```python
from build123d import *

# Parameters (mm, degrees)
SKETCH1_R                = 6
BOSS_EXTRUDE1_DEPTH      = 254
BOSS_EXTRUDE1_DEPTH_BACK = 36
CUT_EXTRUDE3_START       = -36
SKETCH2_W                = 4
SKETCH2_H                = 5
CUT_EXTRUDE3_DEPTH       = 20
CUT_EXTRUDE3_DEPTH_BACK  = 0.0001
CUT_EXTRUDE4_START       = 254
SKETCH2_2_W              = 4
SKETCH2_2_H              = 5
CUT_EXTRUDE4_DEPTH       = 50
CUT_EXTRUDE6_START       = -36
SKETCH3_W                = 4
SKETCH3_H                = 10
CUT_EXTRUDE6_DEPTH       = 6


with BuildPart() as part:
    # Sketch1 → Boss-Extrude1 (new body, two sides)
    with BuildSketch(Plane(origin=(0, 0, 0), x_dir=(1, 0, 0), z_dir=(0, 1, 0))) as boss_extrude1_sk:
        Circle(SKETCH1_R)
    extrude(amount=BOSS_EXTRUDE1_DEPTH)
    extrude(boss_extrude1_sk.sketch, amount=-BOSS_EXTRUDE1_DEPTH_BACK)

    # Sketch2 → Cut-Extrude3 (cut, two sides)
    with BuildSketch(Plane(origin=(0, 0, 0), x_dir=(1, 0, 0), z_dir=(0, 1, 0)).offset(CUT_EXTRUDE3_START)) as cut_extrude3_sk:
        with Locations((0, -6)):
            Rectangle(SKETCH2_W, SKETCH2_H)
    extrude(amount=CUT_EXTRUDE3_DEPTH, mode=Mode.SUBTRACT)
    extrude(cut_extrude3_sk.sketch, amount=-CUT_EXTRUDE3_DEPTH_BACK, mode=Mode.SUBTRACT)

    # Sketch2<2> → Cut-Extrude4 (cut)
    with BuildSketch(Plane(origin=(0, 0, 0), x_dir=(1, 0, 0), z_dir=(0, 1, 0)).offset(CUT_EXTRUDE4_START)):
        with Locations((0, -6)):
            Rectangle(SKETCH2_2_W, SKETCH2_2_H)
    extrude(amount=-CUT_EXTRUDE4_DEPTH, mode=Mode.SUBTRACT)

    # Sketch3 → Cut-Extrude6 (cut)
    with BuildSketch(Plane(origin=(0, 0, 0), x_dir=(1, 0, 0), z_dir=(0, 1, 0)).offset(CUT_EXTRUDE6_START)):
        with Locations((0, -6)):
            Rectangle(SKETCH3_W, SKETCH3_H)
    extrude(amount=CUT_EXTRUDE6_DEPTH, mode=Mode.SUBTRACT)


solid = part.part
```
Geometry check sheet. Reference: the model listing, model coordinates, mm. A direction names the side the tool comes from. Round coordinates to 2 decimals unless told otherwise and drop trailing zeros. Loops run counter-clockwise (first coordinate to the right, second up) from the corner with the lowest first, then second, coordinate; pieces in that order, holes last. Notation, with made-up numbers: (34, 73.5) - (80, 73.5) arc R19 ccw to (80, 96.5) - close; hole circle Ø11 at (37, 14). An arc over 180 degrees is marked (long way). Write each question's results on one line, items separated by ' | '. Start each with the question number.
Q1. Gauge pin test, flat ends, axial feed: P1, Ø1.1, axis at y = 224.5, z = 4, coming from the +X side; P2, Ø3, axis at x = 2.5, y = 34, coming from the -Z side; P3, Ø4.5, axis at x = 0, y = -25, coming from the +Z side. Record the tip position at first contact, or that the pin passes through.
Q2. Release check for a two-part mould opening along X. For faces 1 (the flat face through (2, -28, 4)), 2 (the flat face through (0, -36, 0)), 3 (the cylindrical face through (-0.78, 111.03, -5.95)) record: +X half, -X half, draft (parallel to the pull), parting line (faces both ways), or undercut.
Q3. Cross-section at C-C on y = 127. Enter the section's corners in (x, z), and give its area (3 significant figures).
Q4. Cross-section at A-A on x = 0. Enter the section's corners in (y, z), and give its area (3 significant figures).
Q5. Thickness scan on line 1 (Z direction, x = -0.25, y = 169.5); line 2 (Y direction, x = 0.5, z = 4.75); line 3 (X direction, y = 54.5, z = -0.75). Record the ranges inside material, lowest first. Write a range as [from, to].
Q6. Access from +Z, -Z, +X, -X, +Y, -Y to the whole of each face (thin tool, end or side, straight path). Record for faces 4 (the flat face through (0, 254, 0)), 5 (the flat face through (-2, -28, 4)).
Q7. Cross-section at B-B on y = 206.5. Enter the section's corners in (x, z).
Answers below:
1) P1: stops at x = 4.91 | P2: stops at z = -5.92 | P3: stops at z = 5.66
2) face 1: undercut | face 2: draft | face 3: parting line
3) outline: circle Ø12 at (0, 0) | area: 113 mm²
4) outline: (-36, -6) - (254, -6) - (254, 3.5) - (204, 3.5) - (204, 6) - (-16, 6) - (-16, 3.5) - (-30, 3.5) - (-30, 1) - (-36, 1) - close | area: 3,290 mm²
5) line 1: z = [-5.99, 5.99] | line 2: y = [-16, 204] | line 3: x = [-5.95, 5.95]
6) face 4: +Z, -Z, +X, -X, +Y | face 5: +Z, -Y
7) outline: (-2, 3.5) - (-2, 5.66) arc R6 ccw (long way) to (2, 5.66) - (2, 3.5) - close
